Could you check a few things on this model? Use its own coordinates, in mm. A direction names the side the tool comes from. Round coordinates to 2 decimals unless told otherwise and drop trailing zeros. Order: outer loops, then holes, each group sorted by start corner. A loop starts at its lowest first (then second) coordinate and runs counter-clockwise, first axis right, second up. Notation, with made-up numbers: (66.25, 72.5) -> (96.25, 72.5) arc R22 cw to (96.25, 79.5) -> close; hole circle Ø6 at (1.5, -7.5). An arc over 180 degrees is marked (long way). Put each result on its own line as item: value. Start each with the question number.
Autodesk Inventor part; units mm, degrees
ref_plane "YZ Plane" through (0, 0, 0) normal (1, 0, 0) x (0, 1, 0)
ref_plane "XZ Plane" through (0, 0, 0) normal (0, 1, 0) x (-1, 0, 0)
ref_plane "XY Plane" through (0, 0, 0) normal (0, 0, 1) x (1, 0, 0)
sketch "Sketch1" plane through (0, 0, 0) normal (0, 0, 1) x (1, 0, 0)
  line L0 (-150, 0) -> (150, 0) construction
  line L1 (-150, -35) -> (150, -35)
  line L2 (150, 35) -> (-150, 35)
  arc A0 (-150, 35) -> (-150, -35) centre (-150, 0) ccw
  arc A1 (150, -35) -> (150, 35) centre (150, 0) ccw
  point P0 (0, 0)
  dimension "d0" = 150
  dimension "d1" = 70
extrude "Extrusion1" add sketch "Sketch1" along normal blind 22.5
sketch "Sketch2" plane through (0, 0, 22.5) normal (0, 0, 1) x (1, 0, 0)
  arc A0 (150, -35) -> (150, 35) centre (150, 0) ccw
  line L0 (114, 10) -> (168, 10)
  line L1 (168, 10) -> (168, -10)
  line L2 (168, -10) -> (114, -10)
  line L3 (114, -10) -> (114, 10)
  line L4 (121, 10) -> (161, 10)
  line L5 (161, 10) -> (161, -10)
  line L6 (161, -10) -> (121, -10)
  line L7 (121, -10) -> (121, 10)
  line L8 (114, 0) -> (121, 0)
  line L9 (0, 35) -> (0, -35)
  arc A1 (-150, 35) -> (-150, -35) centre (-150, 0) ccw
  line L10 (-114, 10) -> (-168, 10)
  line L11 (-168, 10) -> (-168, -10)
  line L12 (-168, -10) -> (-114, -10)
  line L13 (-114, -10) -> (-114, 10)
  line L14 (-121, 10) -> (-161, 10)
  line L15 (-161, 10) -> (-161, -10)
  line L16 (-161, -10) -> (-121, -10)
  line L17 (-121, -10) -> (-121, 10)
  line L18 (-114, 0) -> (-121, 0)
  point P0 (0, 0)
  point P1 (168, 0)
  point P2 (121, -10)
  point P3 (161, 10)
  point P4 (-168, 0)
  point P5 (-121, -10)
  point P6 (-161, 10)
  dimension "d4" = 54
  dimension "d5" = 40
  dimension "d6" = 7
  dimension "d7" = 20
  dimension "d8" = 36
extrude "Extrusion2" cut sketch "Sketch2" against normal through all contours L0 L5 L2 L7 | L17 L12 L15 L10
extrude "Extrusion3" cut sketch "Sketch2" against normal blind 13.5 contours L0 L7 L8 L3 | L8 L7 L2 L3 | L0 L1 L2 L5 | L13 L18 L17 L10 | L13 L12 L17 L18 | L15 L12 L11 L10
properties part number "arm 2 right"
1. For pin 1 Ø7 at (y, z) = (5, 4) entering from +X; pin 2 Ø4.5 at (y, z) = (0, 4.5) entering from -X; pin 3 Ø6 at (y, z) = (-22, 14.5) entering from +X, each with a flat end and sliding along its axis, tell me the tip position at first contact or that it passes through.
2. Thinking about a two-plate mould opening in Y: for faces 4 (the face through (141, 10, 11)), 5 (the face through (-2, -35, 11)), 6 (the face through (2, 35, 11)), 7 (the face through (-141, 10, 11)), which applies, +Y half, -Y half, draft (parallel to the pull), parting line (faces both ways), or undercut?
3. If we section it at C-C, the plane y = -22: Please give me the cut outline in (x, z), then the cut area to 3 significant figures.
4. I need wall thicknesses on L1, parallel to X at y = -1.5, z = 3.75; L2, parallel to X at y = -6, z = 9.75; L3, parallel to Y at x = -130, z = 6.5. Which ranges of each line are inside material? Lowest first, please.
5. Which directions (+Z, -Z, +X, -X, +Y, -Y) give clear straight access to the entire face, cutting with the end or side of a thin tool? Please do faces 1 (the face through (114, 0, 16)), 2 (the face through (121, 0, 5)), 3 (the face through (-3, 0, 22.5)).
6. If we section it at B-B, the plane z = 13.25: Please give me the cut outline in (x, y), then the cut area to 3 significant figures.
7. If we section it at A-A, the plane y = 0: Please give me the cut outline in (x, z), then the cut area to 3 significant figures.
Results below:
1. pin 1: x = 184.97
1. pin 2: x = -185
1. pin 3: x = 179.39
2. face 4: undercut
2. face 5: -Y half
2. face 6: +Y half
2. face 7: undercut
3. outline: (-177.22, 0) -> (177.22, 0) -> (177.22, 22.5) -> (-177.22, 22.5) -> close
3. area: 7,970 mm2
4. L1: -184.97 to -161, -121 to 121, 161 to 184.97
4. L2: -184.48 to -168, -114 to 114, 168 to 184.48
4. L3: -35 to -10, 10 to 35
5. face 1: +Z
5. face 2: +Z, -Z
5. face 3: +Z, +X, -X, +Y, -Y
6. outline: (-150, -35) -> (150, -35) arc R35 ccw to (150, 35) -> (-150, 35) arc R35 ccw to start; hole (-168, -10) -> (-114, -10) -> (-114, 10) -> (-168, 10) -> close; hole (114, -10) -> (168, -10) -> (168, 10) -> (114, 10) -> close
6. area: 22,700 mm2
7. outline: (-185, 0) -> (-161, 0) -> (-161, 9) -> (-168, 9) -> (-168, 22.5) -> (-185, 22.5) -> close; (-121, 0) -> (121, 0) -> (121, 9) -> (114, 9) -> (114, 22.5) -> (-114, 22.5) -> (-114, 9) -> (-121, 9) -> close; (161, 0) -> (185, 0) -> (185, 22.5) -> (168, 22.5) -> (168, 9) -> (161, 9) -> close
7. area: 6,150 mm2
